from build123d import *

# Parameters (mm, degrees)
AUFSATZ_LINEAR_AUSTRAGEN1_DEPTH = 3


with BuildPart() as part:
    # Model → Aufsatz-Linear austragen1 (new body)
    with BuildSketch(Plane.XY):
        with BuildLine():
            Line((4, 0), (86, 0))
            ThreePointArc((86, 0), (88.828427125, 1.171572875), (90, 4))
            Line((90, 4), (90, 11))
            ThreePointArc((90, 11), (88.828427125, 13.828427125), (86, 15))
            Line((86, 15), (4, 15))
            ThreePointArc((4, 15), (1.171572875, 13.828427125), (0, 11))
            Line((0, 11), (0, 4))
            ThreePointArc((0, 4), (1.171572875, 1.171572875), (4, 0))
        make_face()
        with BuildLine():
            Line((5, 4.95), (15, 4.95))
            ThreePointArc((15, 4.95), (17.55, 7.5), (15, 10.05))
            Line((15, 10.05), (5, 10.05))
            ThreePointArc((5, 10.05), (2.45, 7.5), (5, 4.95))
        make_face(mode=Mode.SUBTRACT)
        with BuildLine():
            Line((75, 4.95), (85, 4.95))
            ThreePointArc((85, 4.95), (87.55, 7.5), (85, 10.05))
            Line((85, 10.05), (75, 10.05))
            ThreePointArc((75, 10.05), (72.45, 7.5), (75, 4.95))
        make_face(mode=Mode.SUBTRACT)
    extrude(amount=AUFSATZ_LINEAR_AUSTRAGEN1_DEPTH)


solid = part.part
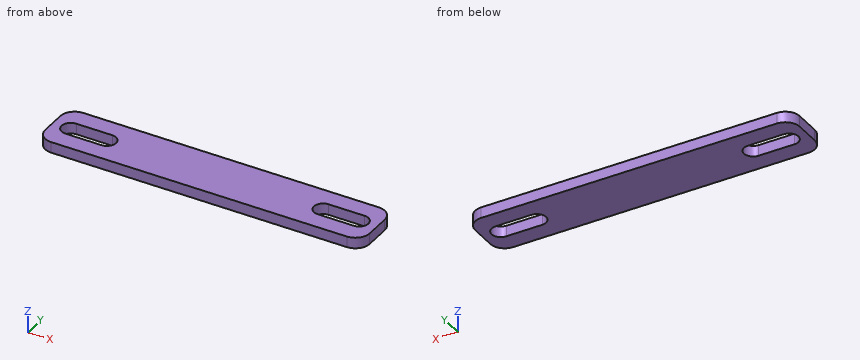
Geometry: final body of the model. Coordinates: model frame, mm. Coordinates: 2 decimals unless noted, no trailing zeros. Order: outer loops, then holes, each group sorted by start corner. A loop starts at its lowest first (then second) coordinate and runs counter-clockwise, first axis right, second up. Notation, with made-up numbers: M 69.25,29 L 126.25,29 A31 cw 126.25,63 Z; hole C 64.25,33 d2. An arc over 180 degrees is marked long. One line per question, with ' | ' between items. Start each with the question number.
Item 1: Ray query, probe 1 along X at (y, z) = (7.75, 2.95); probe 2 along X at (y, z) = (6.5, 0.55); probe 3 along Y at (x, z) = (82, 0.5). Return the intervals inside material, ascending. Write a range as [from, to].
Item 2: Cut plane A-A, the plane x = 11. Return the cut outline in (y, z), then the cut area to 3 significant figures.
Item 3: Cut plane B-B, the plane y = 7.5. Return the cut outline in (x, z), then the cut area to 3 significant figures.
Item 4: Cut plane C-C, the plane z = 2.45. Return the cut outline in (x, y), then the cut area to 3 significant figures.
A:
1) probe 1: x = [0, 2.46], [17.54, 72.46], [87.54, 90] | probe 2: x = [0, 2.65], [17.35, 72.65], [87.35, 90] | probe 3: y = [0, 4.95], [10.05, 15]
2) outline: M 0,0 L 4.95,0 L 4.95,3 L 0,3 Z; M 10.05,0 L 15,0 L 15,3 L 10.05,3 Z | area: 29.7 mm2
3) outline: M 0,0 L 2.45,0 L 2.45,3 L 0,3 Z; M 17.55,0 L 72.45,0 L 72.45,3 L 17.55,3 Z; M 87.55,0 L 90,0 L 90,3 L 87.55,3 Z | area: 179 mm2
4) outline: M 0,4 A4 ccw 4,0 L 86,0 A4 ccw 90,4 L 90,11 A4 ccw 86,15 L 4,15 A4 ccw 0,11 Z; hole M 5,4.95 L 15,4.95 A2.55 ccw 15,10.05 L 5,10.05 A2.55 ccw Z; hole M 75,4.95 L 85,4.95 A2.55 ccw 85,10.05 L 75,10.05 A2.55 ccw Z | area: 1,190 mm2
